from build123d import *

# Parameters (mm, degrees)
SALIENTE_EXTRUIR1_DEPTH = 197
CROQUIS3_W              = 26
CROQUIS3_H              = 22
CORTAR_EXTRUIR1_DEPTH   = 299.793079874


with BuildPart() as part:
    # Croquis1 → Saliente-Extruir1 (new body)
    with BuildSketch(Plane.XY):
        Polygon((219.365853659, 10.012195122), (-50.634146341, 10.012195122), (-50.634146341, -3.987804878), (-54.634146341, -3.987804878), (-54.634146341, -13.987804878), (-49.344908275, -13.987804878), (-46.634146341, -13.987804878), (-46.634146341, -3.987804878), (-46.634146341, 6.012195122), (215.365853659, 6.012195122), (215.365853659, -3.987804878), (215.365853659, -13.987804878), (219.1357706, -13.987804878), (223.365853659, -13.987804878), (223.365853659, -3.987804878), (219.365853659, -3.987804878), align=None)
    extrude(amount=SALIENTE_EXTRUIR1_DEPTH)

    # Croquis3 → Cortar-Extruir1 (cut, through all)
    with BuildSketch(Plane(origin=(0, 10.012195122, 0), x_dir=(1, 0, 0), z_dir=(0, 1, 0))):
        with Locations((-5.684146341, -186)):
            Rectangle(CROQUIS3_W, CROQUIS3_H)
        with Locations((174.415853659, -186)):
            Rectangle(CROQUIS3_W, CROQUIS3_H)
    extrude(amount=-CORTAR_EXTRUIR1_DEPTH, mode=Mode.SUBTRACT)


solid = part.part
Can you work these out from the model? Positions are in its coordinate system, mm. A direction names the side the tool comes from. Round coordinates to 2 decimals unless told otherwise and drop trailing zeros. Write each loop counter-clockwise with the first axis right and the second up, starting at its lowest first coordinate (ties: lowest second). Pieces come first, ordered by that corner, then holes. Notation, with made-up numbers: (-36.75, -25.75) -> (-23.75, -25.75) arc R22 cw to (-23.75, -8.75) -> close; hole circle Ø10 at (70.5, 84). An arc over 180 degrees is marked (long way). Use one line per item in the form item = value. Start each with the question number.
Q1. We'd pull the mould along X, two halves only. Please class faces 1 (the face through (223.366, -9, 97)), 2 (the face through (84, 7, 0)), 3 (the face through (83, 6.012, 97)): +X half, -X half, draft (parallel to the pull), parting line (faces both ways), or undercut.
Q2. Imagine slicing it at B-B (z = 103.5). Please give me the cut outline in (x, y).
Q3. Which directions (+Z, -Z, +X, -X, +Y, -Y) give clear straight access to the entire face, cutting with the end or side of a thin tool? Please do faces 4 (the face through (219.366, 3, 97)), 5 (the face through (86, 10.012, 97)), 6 (the face through (-50.634, 3, 97)), 7 (the face through (-46.634, -4, 97)), 8 (the face through (-51, -13.988, 97)).
Q4. If I drill on probe 1 along X at (y, z) = (-6.75, 180); probe 2 along X at (y, z) = (-0.25, 64.5); probe 3 along Z at (x, y) = (-10, 6.5), over which ranges is the centre line in solid material (lowest first)? Write a range as [from, to].
Q5. I'm going to push flat-ended pins straight in: P1, Ø3, axis at y = 8.5, z = 180.5, coming from the +X side; P2, Ø10, axis at x = 116, z = 111.5, coming from the -Y side; P3, Ø7, axis at y = 1.5, z = 59, coming from the -X side. Where does each tip first touch, or does it pass through?
Q6. Imagine slicing it at C-C (x = -3). Please give me the cut outline in (y, z).
Q7. Imagine slicing it at A-A (y = -7.5). Please give me the cut outline in (x, z), then the cut area to 3 significant figures.
Worked out:
q1.face_1 = +X half
q1.face_2 = draft
q1.face_3 = undercut
q2.outline = (-54.63, -13.99) -> (-46.63, -13.99) -> (-46.63, 6.01) -> (215.37, 6.01) -> (215.37, -13.99) -> (223.37, -13.99) -> (223.37, -3.99) -> (219.37, -3.99) -> (219.37, 10.01) -> (-50.63, 10.01) -> (-50.63, -3.99) -> (-54.63, -3.99) -> close
q3.face_4 = +Z, -Z, +X, +Y
q3.face_5 = +Z, -Z, +X, -X, +Y
q3.face_6 = +Z, -Z, -X, +Y
q3.face_7 = +Z, -Z, -Y
q3.face_8 = +Z, -Z, +X, -X, -Y
q4.probe_1 = [-54.63, -46.63], [215.37, 223.37]
q4.probe_2 = [-50.63, -46.63], [215.37, 219.37]
q4.probe_3 = [0, 175]
q5.P1 = 219.37
q5.P2 = 6.01
q5.P3 = -50.63
q6.outline = (6.01, 0) -> (10.01, 0) -> (10.01, 175) -> (6.01, 175) -> close
q7.outline = (-54.63, 0) -> (-46.63, 0) -> (-46.63, 197) -> (-54.63, 197) -> close; (215.37, 0) -> (223.37, 0) -> (223.37, 197) -> (215.37, 197) -> close
q7.area = 3,150 mm^2
